Drawing for the job (mm, zero at the part's lowest x, y, z). Give positions to 0.01 mm unless a question says otherwise; leave off trailing zeros. Write each loop counter-clockwise with the first axis right and the second up, starting at its lowest first coordinate (ties: lowest second). Pieces come first, ordered by that corner, then holes. Notation, with made-up numbers: M 31,71 L 51,71 A32 ccw 51,108 Z; hole C 14.5,5 d9. An arc over 180 degrees is marked long. Answer as a JSON object with one key per item and string values. Group by question number.
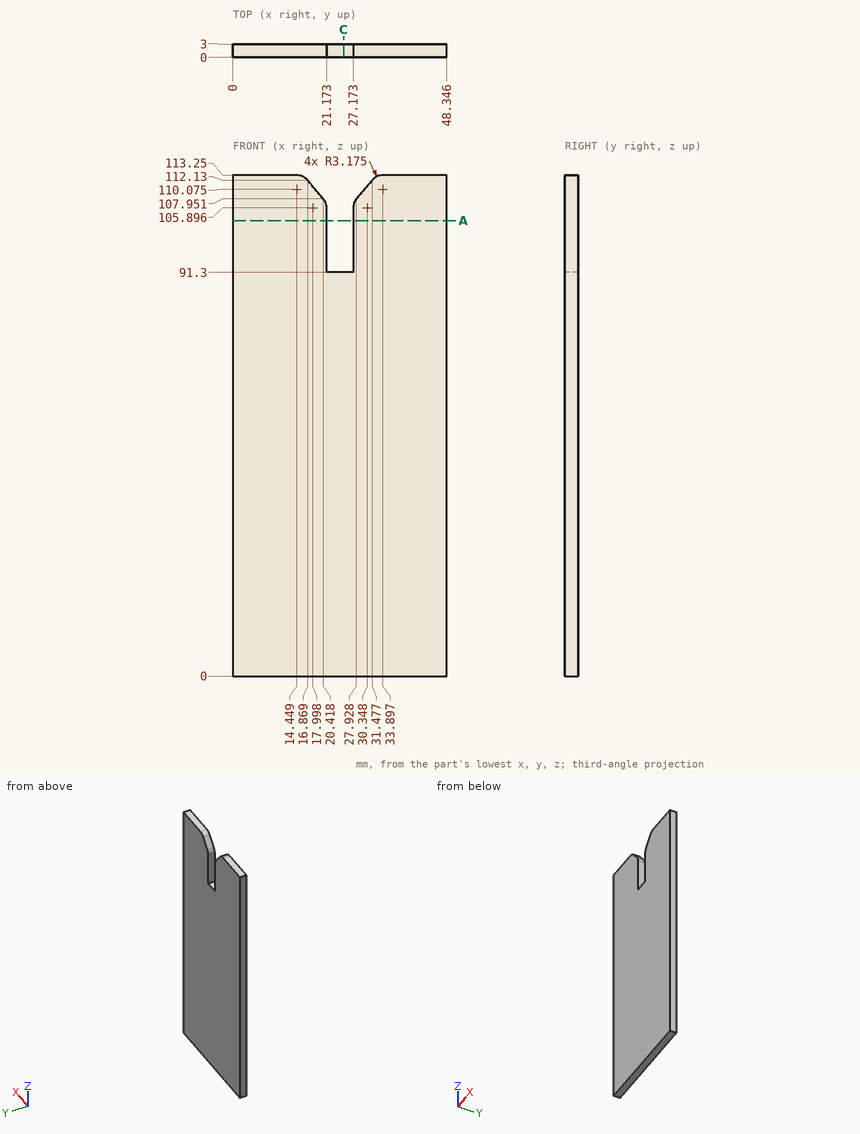
Q1. Wall check: L1, parallel to X at y = 2.5, z = 100.5 (1 decimal); L2, parallel to Z at x = 26.5, y = 2.7; L3, parallel to Z at x = 16, y = 0.15 (1 decimal). Give the ranges that are in metal, low to high.
Q2. Drop a flat-ended pin along its axis: P1, Ø5, axis at x = 24, z = 97.5, coming from the -Y side. Give the stop position or say it passes through.
Q3. Slice it at C-C, the plane x = 25. Write the cut outline in (y, z), then the cut area to 3 significant figures.
Q4. Slice it at A-A, the plane z = 103. Write the cut outline in (x, y) (1 decimal), then the cut area to 3 significant figures.
Solved:
{
 "1": {"L1": "x = 0 to 21.2, 27.2 to 48.3", "L2": "z = 0 to 91.3", "L3": "z = 0 to 112.8"},
 "2": {"P1": "passes through"},
 "3": {"outline": "M 0,0 L 3,0 L 3,91.3 L 0,91.3 Z", "area": "274 mm²"},
 "4": {"outline": "M 0,0 L 21.2,0 L 21.2,3 L 0,3 Z; M 27.2,0 L 48.3,0 L 48.3,3 L 27.2,3 Z", "area": "127 mm²"}
}
